Verification items for the finished model (mm, model axes). Face numbers are marked on the shaded views. A direction names the side the tool comes from. Round coordinates to 2 decimals unless told otherwise and drop trailing zeros. Write each loop counter-clockwise with the first axis right and the second up, starting at its lowest first coordinate (ties: lowest second). Pieces come first, ordered by that corner, then holes. Notation, with made-up numbers: M -39.5,-3 L -34.5,-3 A19 cw -34.5,16 Z; hole C 76,-1 d4. An arc over 180 degrees is marked long. Use a Markdown table: item, result. Add a question column.
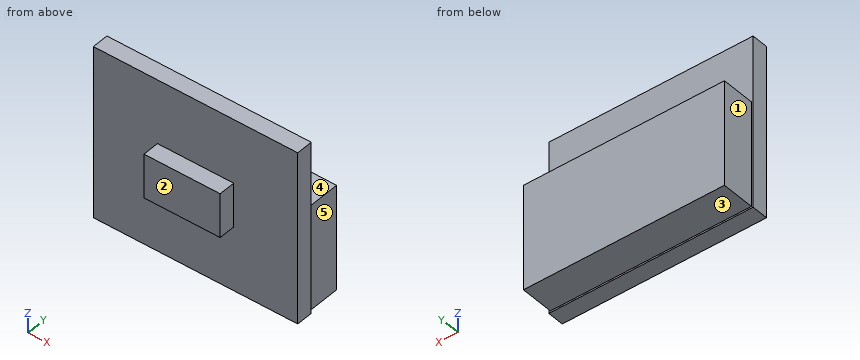
from build123d import *

# Parameters (mm, degrees)
SKETCH1_W           = 12.34
SKETCH1_H           = 10.4
BOSS_EXTRUDE1_DEPTH = 1
SKETCH2_W           = 12.14
SKETCH2_H           = 6.35
BOSS_EXTRUDE2_DEPTH = 2
SKETCH3_W           = 4.6
SKETCH3_H           = 2.66
BOSS_EXTRUDE3_DEPTH = 1


with BuildPart() as part:
    # Sketch1 → Boss-Extrude1 (new body)
    with BuildSketch(Plane(origin=(0, 0, 0), x_dir=(1, 0, 0), z_dir=(0, 1, 0))):
        Rectangle(SKETCH1_W, SKETCH1_H)
    extrude(amount=BOSS_EXTRUDE1_DEPTH)

    # Sketch2 → Boss-Extrude2 (add)
    with BuildSketch(Plane(origin=(0, 1, 0), x_dir=(1, 0, 0), z_dir=(0, 1, 0))):
        with Locations((0, 1.925)):
            Rectangle(SKETCH2_W, SKETCH2_H)
    extrude(amount=BOSS_EXTRUDE2_DEPTH)

    # Sketch3 → Boss-Extrude3 (add)
    with BuildSketch(Plane.XZ):
        Rectangle(SKETCH3_W, SKETCH3_H)
    extrude(amount=BOSS_EXTRUDE3_DEPTH)


solid = part.part
1. Cross-section at C-C on y = -0.35. Enter the section's corners in (x, z), plus the area to 3 significant figures.
2. Cross-section at A-A on x = 0. Enter the section's corners in (y, z).
3. Cross-section at D-D on z = -3.5. Enter the section's corners in (x, y).
4. Cross-section at B-B on z = -0.5. Enter the section's corners in (x, y).
5. Depth check by flat-ended pin: pin 1 Ø0.8 at (x, y) = (-0.5, -0.5) entering from -Z; pin 2 Ø1.6 at (x, y) = (-1, 2) entering from -Z; pin 3 Ø1.6 at (y, z) = (2, -1.5) entering from +X. Enter the tip coordinate at first touch or a pass-through.
6. Scan lines: line 1 along X through (y, z) = (2.25, -0.75); line 2 along Z through (x, y) = (3.5, 1.95); line 3 along Y through (x, z) = (-2.5, 3.5). Record each from-to range of solid material in increasing order. Write a range as from..to.
7. Access from +Z, -Z, +X, -X, +Y, -Y to the whole of each face (thin tool, end or side, straight path). Record for the marked faces 1, 2, 3, 4 and 5.
Answer:
| question | item | result |
|---|---|---|
| 1 | outline | M -2.3,-1.33 L 2.3,-1.33 L 2.3,1.33 L -2.3,1.33 Z |
| 1 | area | 12.2 mm^2 |
| 2 | outline | M -1,-1.33 L 0,-1.33 L 0,-5.2 L 1,-5.2 L 1,-5.1 L 3,-5.1 L 3,1.25 L 1,1.25 L 1,5.2 L 0,5.2 L 0,1.33 L -1,1.33 Z |
| 3 | outline | M -6.17,0 L 6.17,0 L 6.17,1 L 6.07,1 L 6.07,3 L -6.07,3 L -6.07,1 L -6.17,1 Z |
| 4 | outline | M -6.17,0 L -2.3,0 L -2.3,-1 L 2.3,-1 L 2.3,0 L 6.17,0 L 6.17,1 L 6.07,1 L 6.07,3 L -6.07,3 L -6.07,1 L -6.17,1 Z |
| 5 | pin 1 | stops at z = -1.33 |
| 5 | pin 2 | stops at z = -5.1 |
| 5 | pin 3 | stops at x = 6.07 |
| 6 | line 1 | x = -6.07..6.07 |
| 6 | line 2 | z = -5.1..1.25 |
| 6 | line 3 | y = 0..1 |
| 7 | face 1 | +Z, -Z, -X, +Y |
| 7 | face 2 | +Z, -Z, +X, -X, -Y |
| 7 | face 3 | -Z, +X, -X, +Y |
| 7 | face 4 | +Z, +X, -X, +Y |
| 7 | face 5 | +Z, -Z, +X, +Y |
